Check sheet for the modelled part. Datum: model origin and axes. Units: mm. Give positions to 0.01 mm unless a question says otherwise; leave off trailing zeros. Order: outer loops, then holes, each group sorted by start corner. A loop starts at its lowest first (then second) coordinate and runs counter-clockwise, first axis right, second up.
from build123d import *

# Parameters (mm, degrees)
SKETCH_R  = 3.15
PAD_DEPTH = 2.5
FILLET_R  = 5


with BuildPart() as part:
    # Sketch → Pad (new body, symmetric)
    with BuildSketch(Plane.XY):
        Polygon((-250, 15), (15, 15), (15, -175), (-15, -175), (-250, -15), align=None)
        Circle(SKETCH_R, mode=Mode.SUBTRACT)
        with Locations((0, -160)):
            Circle(SKETCH_R, mode=Mode.SUBTRACT)
        with Locations((-30, 0)):
            Circle(SKETCH_R, mode=Mode.SUBTRACT)
        with Locations((-235, 0)):
            Circle(SKETCH_R, mode=Mode.SUBTRACT)
    extrude(amount=PAD_DEPTH, both=True)

    # Fillet
    fillet_edges = [part.edges().sort_by_distance(p)[0] for p in [
        (-250, 15, 0),
        (-250, -15, 0),
        (15, 15, 0),
        (-15, -175, 0),
        (15, -175, 0),
    ]]
    fillet(fillet_edges, radius=FILLET_R)


solid = part.part
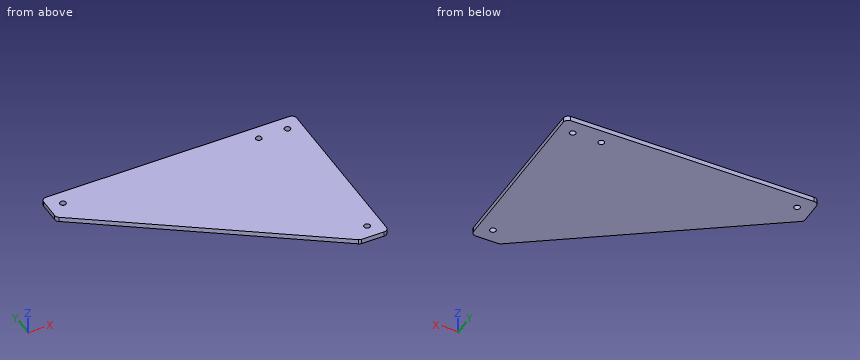
1) Material ranges on L1, parallel to Y at x = 0, z = 0.3; L2, parallel to Y at x = -235, z = 0.3; L3, parallel to Y at x = -30, z = -1, recorded low to high.
Recorded:
L1: y = -175 to -163.15, -156.85 to -3.15, 3.15 to 15
L2: y = -25.21 to -3.15, 3.15 to 15
L3: y = -164.79 to -3.15, 3.15 to 15
2) Section check A-A, the plane x = 0. Record the cut outline in (y, z).
Recorded:
outline: (-175, -2.5) - (-163.15, -2.5) - (-163.15, 2.5) - (-175, 2.5) - close; (-156.85, -2.5) - (-3.15, -2.5) - (-3.15, 2.5) - (-156.85, 2.5) - close; (3.15, -2.5) - (15, -2.5) - (15, 2.5) - (3.15, 2.5) - close
3) Section check B-B, the plane y = 0. Record the cut outline in (x, z), then the cut area to 3 significant figures.
Recorded:
outline: (-250, -2.5) - (-238.15, -2.5) - (-238.15, 2.5) - (-250, 2.5) - close; (-231.85, -2.5) - (-33.15, -2.5) - (-33.15, 2.5) - (-231.85, 2.5) - close; (-26.85, -2.5) - (-3.15, -2.5) - (-3.15, 2.5) - (-26.85, 2.5) - close; (3.15, -2.5) - (15, -2.5) - (15, 2.5) - (3.15, 2.5) - close
area: 1,230 mm2
4) Section check D-D, the plane x = -30. Record the cut outline in (y, z).
Recorded:
outline: (-164.79, -2.5) - (-3.15, -2.5) - (-3.15, 2.5) - (-164.79, 2.5) - close; (3.15, -2.5) - (15, -2.5) - (15, 2.5) - (3.15, 2.5) - close
5) Section check C-C, the plane z = -1.65. Record the cut outline in (x, y).
Recorded:
outline: (-250, -12.36) arc R5 ccw to (-247.81, -16.49) - (-16.27, -174.13) arc R5 ccw to (-13.46, -175) - (10, -175) arc R5 ccw to (15, -170) - (15, 10) arc R5 ccw to (10, 15) - (-245, 15) arc R5 ccw to (-250, 10) - close; hole circle Ø6.3 at (-235, 0); hole circle Ø6.3 at (-30, 0); hole circle Ø6.3 at (0, -160); hole circle Ø6.3 at (0, 0)
